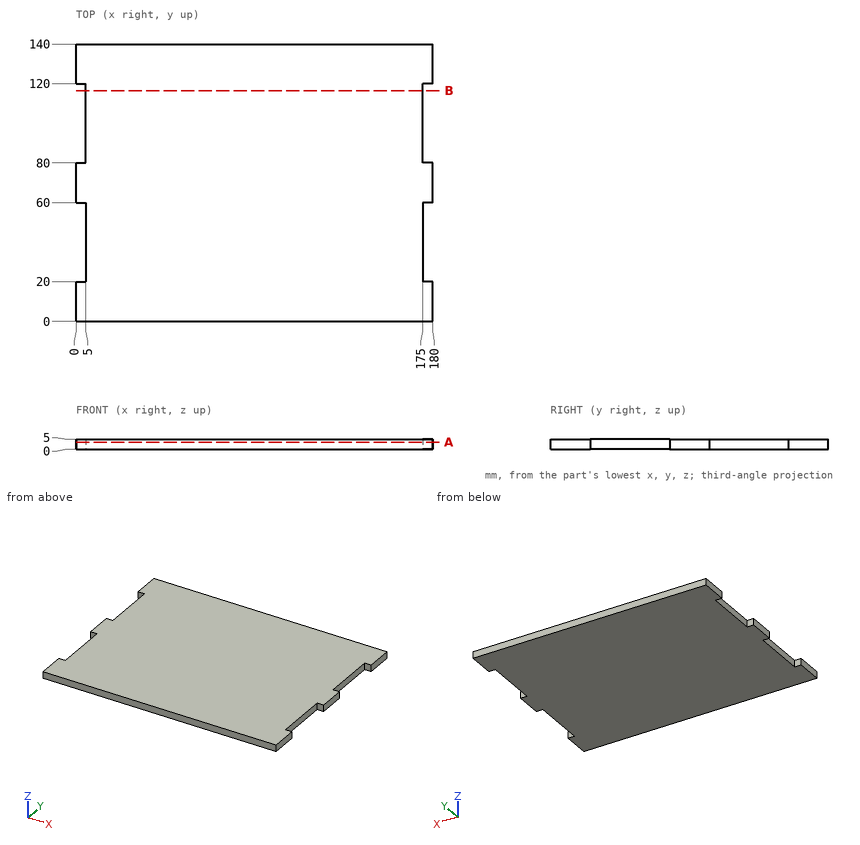
Check sheet for the drawn part. Datum: minimum x, y, z corner. Units: mm. Give positions to 0.01 mm unless a question says otherwise; leave off trailing zeros. Order: outer loops, then holes, each group sorted by start corner. A loop starts at its lowest first (then second) coordinate and runs counter-clockwise, first axis right, second up. Notation, with made-up numbers: (-28, -5.75) -> (24, -5.75) arc R19 cw to (24, 10.25) -> close; hole circle Ø3 at (-30.5, -6.75). An arc over 180 degrees is marked (long way). Use a Markdown table: item, result.
1) Material ranges on probe 1 along X at (y, z) = (44, 2.05), recorded low to high.
Results:
| item | result |
|---|---|
| probe 1 | 5 to 175 |
2) Section check A-A, the plane z = 3.65. Record the boundary of the cut face in (x, y), then the cut area to 3 significant figures.
Results:
| item | result |
|---|---|
| outline | (0, 0) -> (180, 0) -> (180, 20) -> (175, 20) -> (175, 60) -> (180, 60) -> (180, 80) -> (175, 80) -> (175, 120) -> (180, 120) -> (180, 140) -> (0, 140) -> (0, 120) -> (5, 120) -> (5, 80) -> (0, 80) -> (0, 60) -> (5, 60) -> (5, 20) -> (0, 20) -> close |
| area | 24,400 mm² |
3) Section check B-B, the plane y = 116.5. Record the boundary of the cut face in (x, z).
Results:
| item | result |
|---|---|
| outline | (5, 0) -> (175, 0) -> (175, 5) -> (5, 5) -> close |
4) Depth check by flat-ended pin: pin 1 Ø1.5 at (y, z) = (107.5, 3.5) entering from -X. Enter the tip coordinate at first touch or a pass-through.
Results:
| item | result |
|---|---|
| pin 1 | x = 5 |
